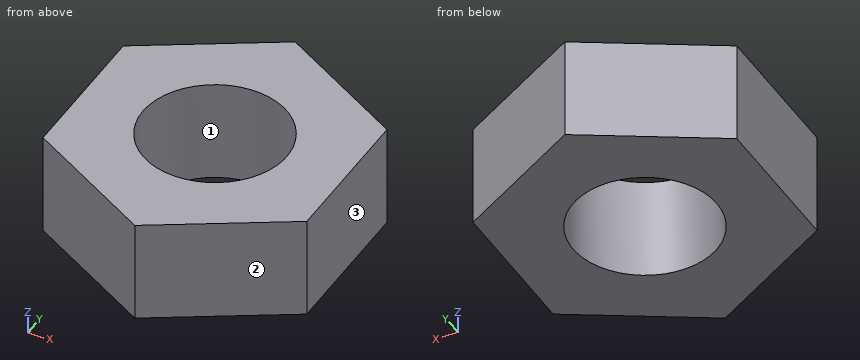
from build123d import *

# Parameters (mm, degrees)
BOSS_EXTRUDE1_DEPTH         = 3
TAP_DRILL_FOR_M5X0_8_TAP1_D = 4.2


with BuildPart() as part:
    # Sketch1 → Boss-Extrude1 (new body)
    with BuildSketch(Plane(origin=(0, 0, 0), x_dir=(0, 1, 0), z_dir=(0, 0, 1))):
        Polygon((-4.445597073, 0), (-2.222798536, -3.85), (2.222798536, -3.85), (4.445597073, 0), (2.222798536, 3.85), (-2.222798536, 3.85), align=None)
    extrude(amount=BOSS_EXTRUDE1_DEPTH)

    # Tap Drill for M5x0.8 Tap1 (through all)
    with Locations(Plane.XY.offset(3)):
        with Locations((0, 0)):
            Hole(TAP_DRILL_FOR_M5X0_8_TAP1_D / 2)


solid = part.part
Can you work these out from the model? Positions are in its coordinate system, mm. Face numbers are marked on the shaded views. Coordinates: 2 decimals unless noted, no trailing zeros. Loops run counter-clockwise (first coordinate to the right, second up) from the corner with the lowest first, then second, coordinate; pieces in that order, holes last. Notation, with made-up numbers: M -4,29 L 20,29 A15 cw 20,45 Z; hole C -23,-14 d11. An arc over 180 degrees is marked long. Answer as CSV lines item,"result". Start each with the question number.
1. Suppose I cut it at A-A, the plane y = 0. List the corners of the cut face in (x, z) for me, plus the area to 3 significant figures.
2. Thinking about a two-plate mould opening in Y: for the marked faces 1, 2 and 3, which applies, +Y half, -Y half, draft (parallel to the pull), parting line (faces both ways), or undercut?
3. Suppose I cut it at B-B, the plane z = 0.3. List the corners of the cut face in (x, y) for me.
4. If I drill on probe 1 along Y at (x, z) = (1.25, 2.7); probe 2 along Y at (x, z) = (-0.75, 1.3); probe 3 along X at (y, z) = (0.25, 1.15), over which ranges is the centre line in solid material (lowest first)? Write a range as [from, to].
5. Suppose I cut it at D-D, the plane x = 3. List the corners of the cut face in (y, z) for me, plus the area to 3 significant figures.
6. For pin 1 Ø4 at (x, y) = (1, 0.5) entering from +Z; pin 2 Ø1.5 at (x, z) = (-3, 1) entering from -Y, each with a flat end and sliding along its axis, tell me the tip position at first contact or that it passes through.
7. Suppose I cut it at C-C, the plane x = 0.25. List the corners of the cut face in (y, z) for me, plus the area to 3 significant figures.
Output:
1,outline,"M -3.85,0 L -2.1,0 L -2.1,3 L -3.85,3 Z; M 2.1,0 L 3.85,0 L 3.85,3 L 2.1,3 Z"
1,area,"10.5 mm^2"
2,face 1,"undercut"
2,face 2,"-Y half"
2,face 3,"draft"
3,outline,"M -3.85,-2.22 L 0,-4.45 L 3.85,-2.22 L 3.85,2.22 L 0,4.45 L -3.85,2.22 Z; hole C 0,0 d4.2"
4,probe 1,"y = [-3.72, -1.69], [1.69, 3.72]"
4,probe 2,"y = [-4.01, -1.96], [1.96, 4.01]"
4,probe 3,"x = [-3.85, -2.09], [2.09, 3.85]"
5,outline,"M -2.71,0 L 2.71,0 L 2.71,3 L -2.71,3 Z"
5,area,"16.3 mm^2"
6,pin 1,"stops at z = 3"
6,pin 2,"stops at y = -3.15"
7,outline,"M -4.3,0 L -2.09,0 L -2.09,3 L -4.3,3 Z; M 2.09,0 L 4.3,0 L 4.3,3 L 2.09,3 Z"
7,area,"13.3 mm^2"
